Can you work these out from the drawing? Everything is in mm from the part's minimum corner. Coordinates: 2 decimals unless noted, no trailing zeros. Write each loop counter-clockwise with the first axis right and the second up, starting at its lowest first coordinate (ties: lowest second). Pieces come first, ordered by that corner, then holes. Notation, with made-up numbers: M 3,-5 L 37,-5 A16 cw 37,24 Z; hole C 26.25,-37.5 d10. An arc over 180 degrees is marked long. Write item = value, one per line.
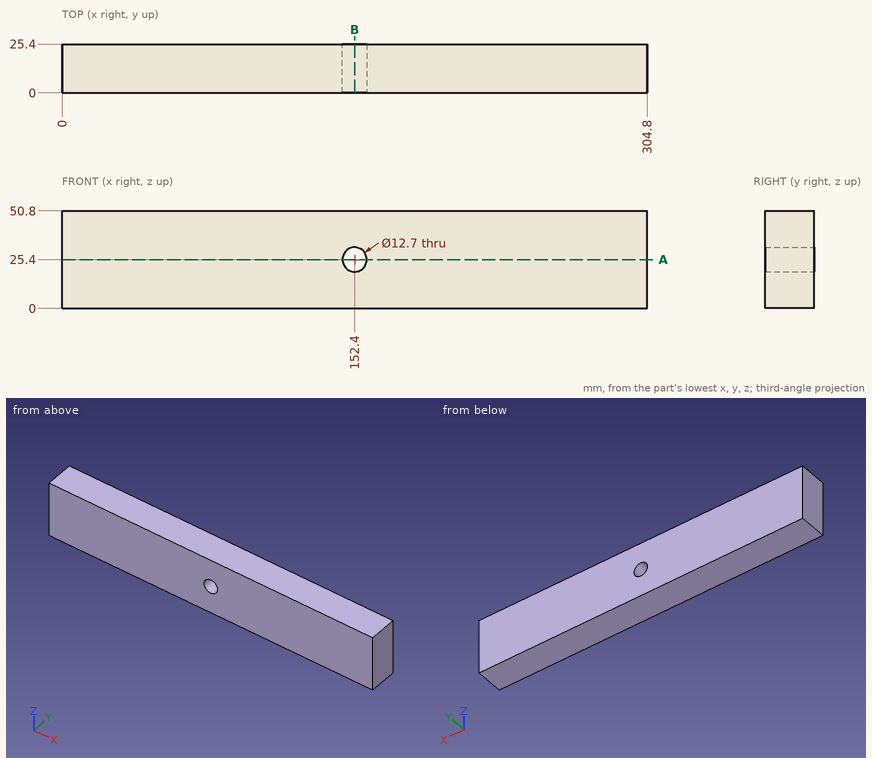
Item 1: Imagine slicing it at A-A (z = 25.4). Write out the boundary of the cut face in (x, y), and give its area (3 significant figures).
Numbers:
outline = M 0,0 L 146.05,0 L 146.05,25.4 L 0,25.4 Z; M 158.75,0 L 304.8,0 L 304.8,25.4 L 158.75,25.4 Z
area = 7,420 mm²
Item 2: Imagine slicing it at B-B (x = 152.4). Write out the boundary of the cut face in (y, z), and give its area (3 significant figures).
Numbers:
outline = M 0,0 L 25.4,0 L 25.4,19.05 L 0,19.05 Z; M 0,31.75 L 25.4,31.75 L 25.4,50.8 L 0,50.8 Z
area = 968 mm²
Item 3: If I drill on line 1 along Z through (x, y) = (152.4, 7); line 2 along X through (y, z) = (22.5, 21); line 3 along X through (y, z) = (10.5, 22), over which ranges is the centre line in solid material (lowest first)?
Numbers:
line_1 = 0 to 19.05, 31.75 to 50.8
line_2 = 0 to 147.82, 156.98 to 304.8
line_3 = 0 to 147.04, 157.76 to 304.8
